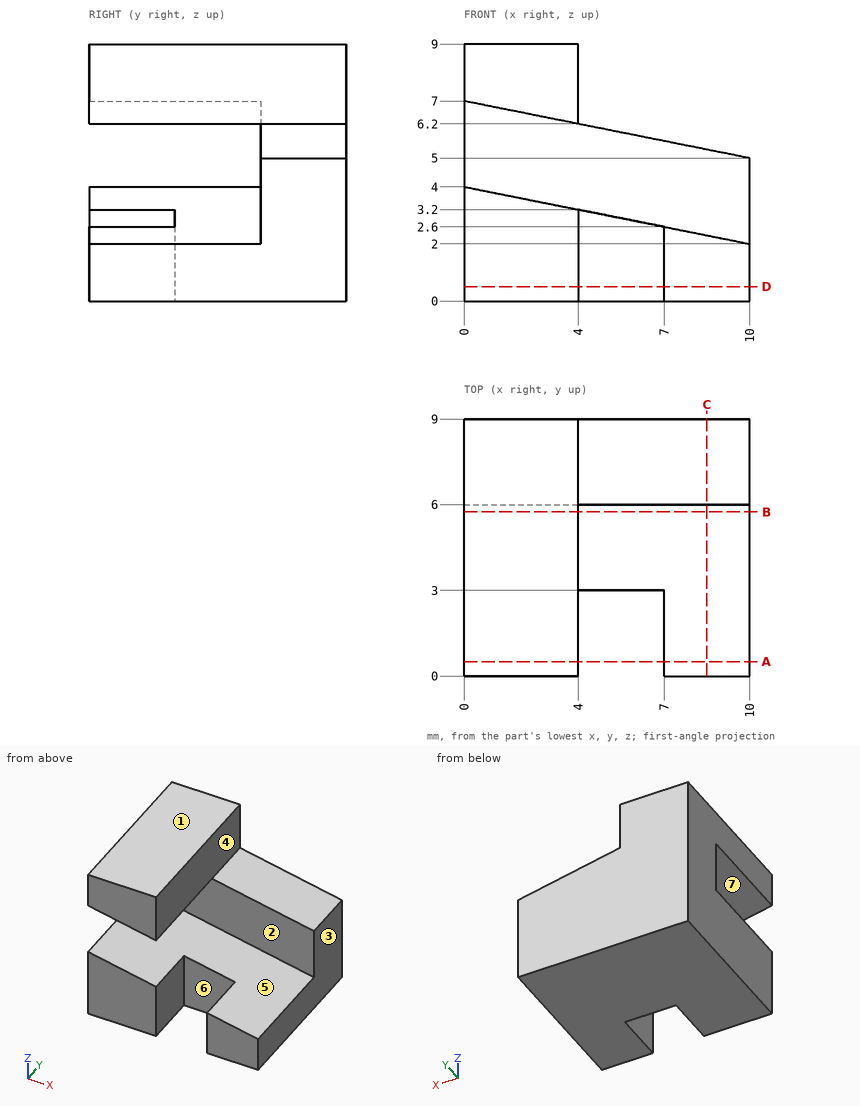
Check sheet for the drawn part. Datum: minimum x, y, z corner. Units: mm. A direction names the side the tool comes from. Give positions to 0.01 mm unless a question says otherwise; leave off trailing zeros. Order: outer loops, then holes, each group sorted by start corner. A loop starts at its lowest first (then second) coordinate and runs counter-clockwise, first axis right, second up. Notation, with made-up numbers: (77, -2.5) -> (109, -2.5) arc R24 ccw to (109, 22.5) -> close; hole circle Ø10 at (42, -8.5). An arc over 180 degrees is marked (long way). One line per item, written item: value.
(1) Draft check along Z on the marked faces 1, 2 and 3. Enter one of: pulls with the +Z half, pulls with the -Z half, needs draft (parallel to the pull), parting line crosses it, or undercut.
Final values:
face 1: pulls with the +Z half
face 2: undercut
face 3: needs draft
(2) Tool access check on the marked faces 4, 5, 6 and 7. Record the directions out of +Z, -Z, +X, -X, +Y, -Y that give a thin tool (end or side, any length) a straight path to the whole face; none if there is none.
Final values:
face 4: +Z, +X, +Y, -Y
face 5: +X, -Y
face 6: +Z, -Z, -Y
face 7: -X, -Y
(3) Sectioned sample at B-B on y = 5.75. Record the cut outline in (x, z).
Final values:
outline: (0, 0) -> (10, 0) -> (10, 2) -> (0, 4) -> close; (0, 7) -> (4, 6.2) -> (4, 9) -> (0, 9) -> close
(4) Sectioned sample at D-D on z = 0.5. Record the cut outline in (x, y).
Final values:
outline: (0, 0) -> (4, 0) -> (4, 3) -> (7, 3) -> (7, 0) -> (10, 0) -> (10, 9) -> (0, 9) -> close
(5) Scan lines: line 1 along X through (y, z) = (0.75, 3); line 2 along Y through (x, z) = (0.75, 4.25); line 3 along X through (y, z) = (2.25, 1.5). Record each from-to range of solid material in increasing order. Write a range as [from, to].
Final values:
line 1: [0, 4]
line 2: [6, 9]
line 3: [0, 4], [7, 10]
(6) Sectioned sample at A-A on y = 0.5. Record the cut outline in (x, z).
Final values:
outline: (0, 0) -> (4, 0) -> (4, 3.2) -> (0, 4) -> close; (0, 7) -> (4, 6.2) -> (4, 9) -> (0, 9) -> close; (7, 0) -> (10, 0) -> (10, 2) -> (7, 2.6) -> close
(7) Gauge pin test, flat ends, axial feed: pin 1 (0.8 mm diameter, centred on y = 6.5, z = 7.5, fed in from +X); pin 2 (5 mm diameter, centred on x = 2.5, y = 4.5, fed in from -Z); pin 3 (1.5 mm diameter, centred on x = 5.5, z = 2, fed in from -Y); pin 4 (2.5 mm diameter, centred on x = 5.5, z = 5, fed in from -Y). Record the tip position at first contact, or that the pin passes through.
Final values:
pin 1: x = 4
pin 2: z = 0
pin 3: y = 3
pin 4: y = 6
(8) Sectioned sample at C-C on x = 8.5. Record the cut outline in (y, z), then the cut area to 3 significant figures.
Final values:
outline: (0, 0) -> (9, 0) -> (9, 5.3) -> (6, 5.3) -> (6, 2.3) -> (0, 2.3) -> close
area: 29.7 mm^2
